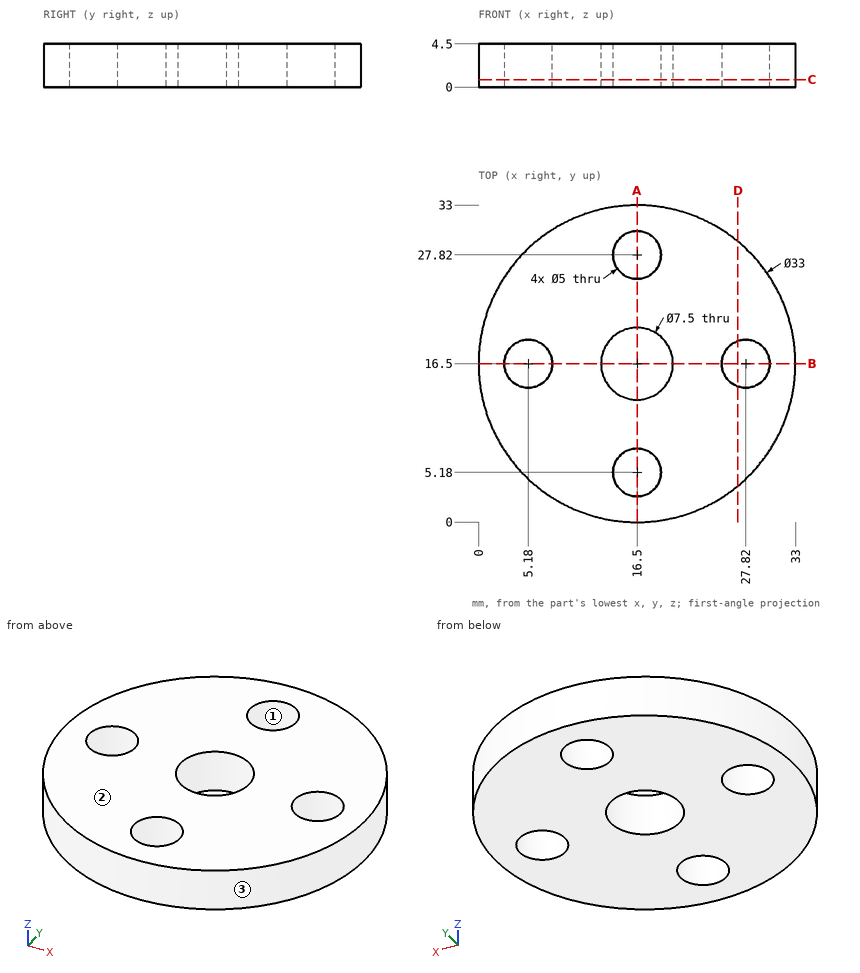
Part print with two shaded views. Sizes in mm from the minimum x, y, z corner. Coordinates: 2 decimals unless noted, no trailing zeros. Write each loop counter-clockwise with the first axis right and the second up, starting at its lowest first coordinate (ties: lowest second). Pieces come first, ordered by that corner, then holes. Notation, with made-up numbers: (77, 15) - (118, 15) arc R22 ccw to (118, 34) - close; hole circle Ø7 at (51.25, 52.5). An arc over 180 degrees is marked (long way). Use a Markdown table: item, result. Add a question column.
Item 1: Two-plate mould, pull along X, no slides. Class the marked faces 1, 2 and 3: pulls with the +X half, pulls with the -X half, needs draft (parallel to the pull), parting line crosses it, or undercut.
Item 2: Drill centre lines: line 1 along Y through (x, z) = (16.5, 3.1); line 2 along Y through (x, z) = (27.82, 3.2); line 3 along Y through (x, z) = (17.5, 3.1). Where is each one in solid material? Low to high.
Item 3: Band-saw the part on A-A, the plane x = 16.5. Write the cut outline in (y, z), and give its area (4 significant figures).
Item 4: Drop flat-ended pins along their axis: pin 1 (1 mm diameter, centred on y = 10, z = 4, fed in from +X); pin 2 (1 mm diameter, centred on x = 6, z = 3, fed in from +Y). Give the stop position or say it passes through.
Item 5: Band-saw the part on C-C, the plane z = 0.8. Write the cut outline in (x, y), and give its area (3 significant figures).
Item 6: Band-saw the part on D-D, the plane x = 27. Write the cut outline in (y, z).
A:
| question | item | result |
|---|---|---|
| 1 | face 1 | undercut |
| 1 | face 2 | needs draft |
| 1 | face 3 | parting line crosses it |
| 2 | line 1 | y = 0 to 2.68, 7.68 to 12.75, 20.25 to 25.32, 30.32 to 33 |
| 2 | line 2 | y = 4.5 to 14, 19 to 28.5 |
| 2 | line 3 | y = 0.03 to 2.89, 7.47 to 12.89, 20.11 to 25.53, 30.11 to 32.97 |
| 3 | outline | (0, 0) - (2.68, 0) - (2.68, 4.5) - (0, 4.5) - close; (7.68, 0) - (12.75, 0) - (12.75, 4.5) - (7.68, 4.5) - close; (20.25, 0) - (25.32, 0) - (25.32, 4.5) - (20.25, 4.5) - close; (30.32, 0) - (33, 0) - (33, 4.5) - (30.32, 4.5) - close |
| 3 | area | 69.75 mm² |
| 4 | pin 1 | stops at x = 31.87 |
| 4 | pin 2 | stops at y = 29.62 |
| 5 | outline | circle Ø33 at (16.5, 16.5); hole circle Ø5 at (5.18, 16.5); hole circle Ø7.5 at (16.5, 16.5); hole circle Ø5 at (16.5, 5.18); hole circle Ø5 at (16.5, 27.82); hole circle Ø5 at (27.82, 16.5) |
| 5 | area | 733 mm² |
| 6 | outline | (3.77, 0) - (14.14, 0) - (14.14, 4.5) - (3.77, 4.5) - close; (18.86, 0) - (29.23, 0) - (29.23, 4.5) - (18.86, 4.5) - close |
